```python
from build123d import *

# Parameters (mm, degrees)
TAGLIO_ESTRUSIONE1_DEPTH      = 6.629165125
TAGLIO_ESTRUSIONE1_DEPTH_BACK = 6.629165125
SCHIZZO2_R                    = 1.46
TAGLIO_ESTRUSIONE2_DEPTH      = 6.436533822
TAGLIO_ESTRUSIONE2_DEPTH_BACK = 6.436533822
SCHIZZO3_W                    = 0.403601212
SCHIZZO3_H                    = 6.501424145


with BuildPart() as part:
    # Schizzo1 → Rivoluzione1 (revolve)
    with BuildSketch(Plane.XY):
        with BuildLine():
            Line((0, 3.25), (0, -3.25))
            ThreePointArc((0, -3.25), (3.25, 0), (0, 3.25))
        make_face()
    revolve(axis=Axis((0, 3.25, 0), (0, -1, 0)))

    # Schizzo2 → Taglio-Estrusione1 (cut, two sides: drawn at the far end of the back side and taken through both)
    with BuildSketch(Plane(origin=(0, 0, 0), x_dir=(0, 0, -1), z_dir=(1, 0, 0)).offset(-TAGLIO_ESTRUSIONE1_DEPTH_BACK)):
        with Locations(Location((0, 0, 0), (0, 0, 180))):
            Circle(SCHIZZO2_R)
    extrude(amount=TAGLIO_ESTRUSIONE1_DEPTH + TAGLIO_ESTRUSIONE1_DEPTH_BACK, mode=Mode.SUBTRACT)

    # Schizzo3 → Taglio-Estrusione2 (cut, two sides: drawn at the far end of the back side and taken through both)
    with BuildSketch(Plane.XY.offset(-TAGLIO_ESTRUSIONE2_DEPTH_BACK)):
        with Locations((2.701800606, 0.000712073)):
            Rectangle(SCHIZZO3_W, SCHIZZO3_H)
        with Locations((-2.701800606, 0.000712073)):
            Rectangle(SCHIZZO3_W, SCHIZZO3_H)
    extrude(amount=TAGLIO_ESTRUSIONE2_DEPTH + TAGLIO_ESTRUSIONE2_DEPTH_BACK, mode=Mode.SUBTRACT)


solid = part.part
```
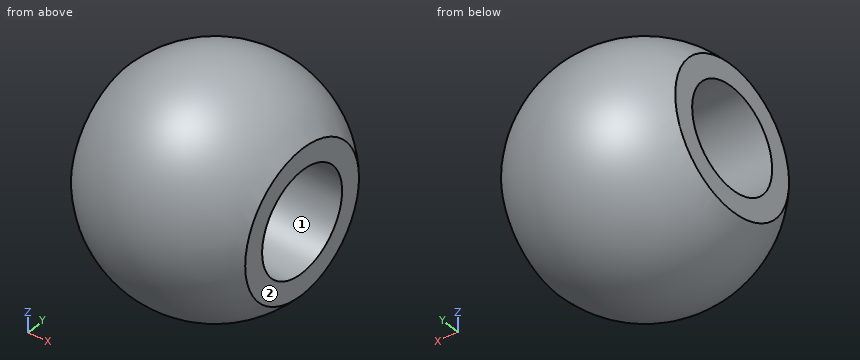
For this review, take the finished solid that the model builds, in its own axes (mm). Face numbers are marked on the shaded views. Round coordinates to 2 decimals unless told otherwise and drop trailing zeros. Write each loop counter-clockwise with the first axis right and the second up, starting at its lowest first coordinate (ties: lowest second). Pieces come first, ordered by that corner, then holes. Notation, with made-up numbers: (-17.75, 62.25) - (14.25, 62.25) arc R23 cw to (14.25, 78.25) - close; hole circle Ø2 at (33, 60.5). An arc over 180 degrees is marked (long way). Answer as a JSON object with one key per item and string values.
1. We need section C-C on x = 0.65. Give the boundary of the cut face in (y, z), then the cut area to 3 significant figures.
Response values:
{"outline": "circle Ø6.37 at (0, 0); hole circle Ø2.92 at (0, 0)", "area": "25.2 mm2"}
2. We need section A-A on z = 0. Give the boundary of the cut face in (x, y).
Response values:
{"outline": "(-2.5, -2.08) arc R3.25 ccw to (2.5, -2.08) - (2.5, -1.46) - (-2.5, -1.46) - close; (-2.5, 1.46) - (2.5, 1.46) - (2.5, 2.08) arc R3.25 ccw to (-2.5, 2.08) - close"}
3. For pin 1 Ø2 at (x, y) = (0, -2) entering from -Z; pin 2 Ø1.5 at (x, z) = (0.5, -2) entering from +Y, all flat-tipped, find the tip position at first contact; note any pin that passes through.
Response values:
{"pin 1": "stops at z = -3.09", "pin 2": "stops at y = 2.97"}
4. We need section D-D on z = 2.25. Give the boundary of the cut face in (x, y), then the cut area to 3 significant figures.
Response values:
{"outline": "circle Ø4.69 at (0, 0)", "area": "17.3 mm2"}
5. Draft analysis for pull direction Y (two halves, no side actions). For the marked faces 1 and 2, state which applies: +Y half, -Y half, draft (parallel to the pull), parting line (faces both ways), or undercut.
Response values:
{"face 1": "undercut", "face 2": "draft"}
6. To check wall thickness, follow line 1 along Y through (x, z) = (0.9, -0.75); line 2 along Y through (x, z) = (-0.2, 0); line 3 along Z through (x, y) = (-0.7, -0.5). State the ranges of each line that lie inside material, in increasing order.
Response values:
{"line 1": "y = -3.03 to -1.25, 1.25 to 3.03", "line 2": "y = -3.24 to -1.46, 1.46 to 3.24", "line 3": "z = -3.13 to -1.37, 1.37 to 3.13"}
